For this review, use the dimensioned drawing (mm, ordinates from the lowest corner) and the shaded views. A direction names the side the tool comes from. Coordinates: 2 decimals unless noted, no trailing zeros. Loops run counter-clockwise (first coordinate to the right, second up) from the corner with the lowest first, then second, coordinate; pieces in that order, holes last. Notation, with made-up numbers: (-14, 67.25) - (26, 67.25) arc R27 cw to (26, 88.25) - close; hole circle Ø1 at (58, 71.25). An arc over 180 degrees is marked (long way). Answer in a Markdown table with one row per item. Add a question column.
(1) Mouldability with a two-part tool opening along Z and no side actions: class the marked faces 1, 2 and 3 as +Z half, -Z half, draft (parallel to the pull), parting line (faces both ways), or undercut.
(2) We need section B-B on x = 19.45. Write out the cut boundary in (y, z), plus the area to 3 significant figures.
(3) Machinability: for the marked faces 4, 5 and 6, which of the approach directions +Z, -Z, +X, -X, +Y, -Y give a long, thin tool a straight path to every point of the face, cutting with its end or side? Answer none if there is none.
(4) We need section C-C on z = 17.5. Write out the cut boundary in (x, y), plus the area to 3 significant figures.
(5) For P1, Ø1.7, axis at x = 10, z = 17.5, coming from the +Y side; P2, Ø10, axis at x = 24, z = 12, coming from the -Y side, all flat-tipped, find the tip position at first contact; note any pin that passes through.
(6) For line 1 along X through (y, z) = (4.5, 17.5); line 2 along Z through (x, y) = (3, 3.5); line 3 along Z through (x, y) = (9.75, 4), list the stretches that pass through material, from the lowest coordinate up.
(7) We need section D-D on x = 5.5. Write out the cut boundary in (y, z).
(8) We need section A-A on y = 5.25. Write out the cut boundary in (x, z), plus the area to 3 significant figures.
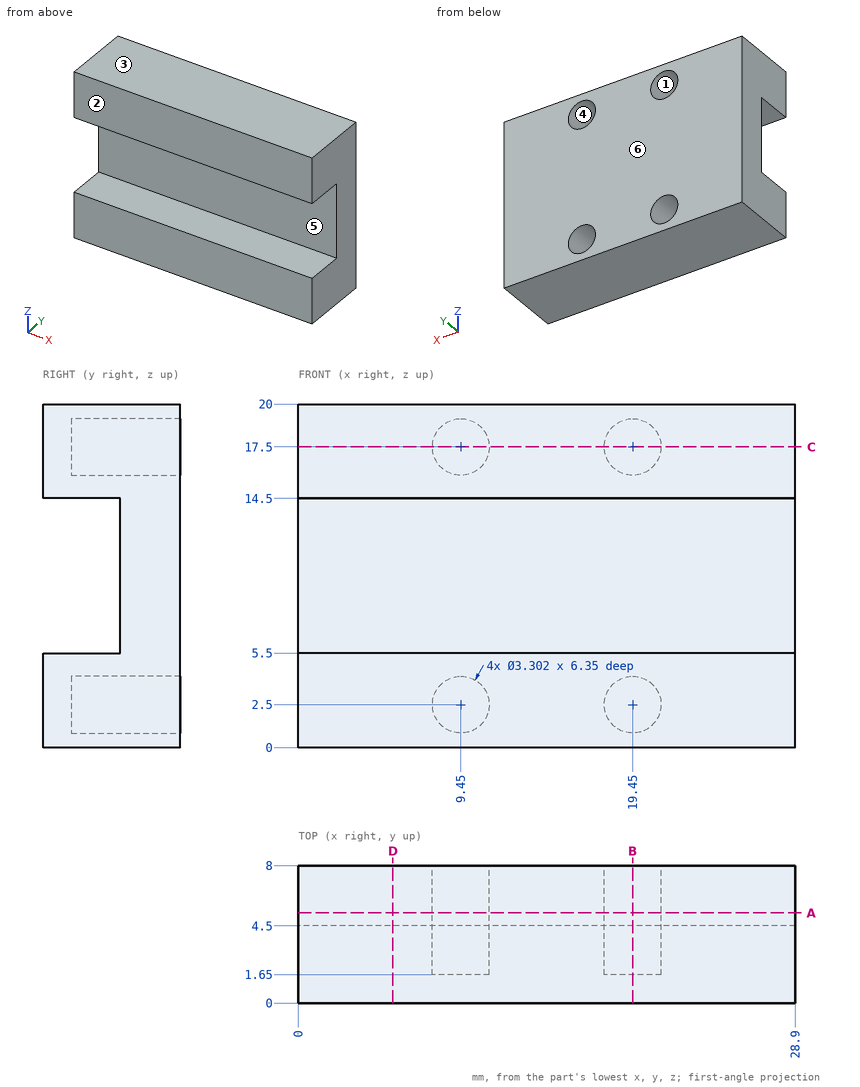
Outcome:
| question | item | result |
|---|---|---|
| 1 | face 1 | undercut |
| 1 | face 2 | draft |
| 1 | face 3 | +Z half |
| 2 | outline | (0, 0) - (8, 0) - (8, 0.85) - (1.65, 0.85) - (1.65, 4.15) - (8, 4.15) - (8, 15.85) - (1.65, 15.85) - (1.65, 19.15) - (8, 19.15) - (8, 20) - (0, 20) - (0, 14.5) - (4.5, 14.5) - (4.5, 5.5) - (0, 5.5) - close |
| 2 | area | 77.6 mm² |
| 3 | face 4 | +Y |
| 3 | face 5 | +X, -X, -Y |
| 3 | face 6 | +Z, -Z, +X, -X, +Y |
| 4 | outline | (0, 0) - (28.9, 0) - (28.9, 8) - (21.1, 8) - (21.1, 1.65) - (17.8, 1.65) - (17.8, 8) - (11.1, 8) - (11.1, 1.65) - (7.8, 1.65) - (7.8, 8) - (0, 8) - close |
| 4 | area | 189 mm² |
| 5 | P1 | y = 1.65 |
| 5 | P2 | y = 0 |
| 6 | line 1 | 0 to 7.8, 11.1 to 17.8, 21.1 to 28.9 |
| 6 | line 2 | 0 to 5.5, 14.5 to 20 |
| 6 | line 3 | 0 to 0.88, 4.12 to 5.5, 14.5 to 15.88, 19.12 to 20 |
| 7 | outline | (0, 0) - (8, 0) - (8, 20) - (0, 20) - (0, 14.5) - (4.5, 14.5) - (4.5, 5.5) - (0, 5.5) - close |
| 8 | outline | (0, 0) - (28.9, 0) - (28.9, 20) - (0, 20) - close; hole circle Ø3.3 at (9.45, 2.5); hole circle Ø3.3 at (9.45, 17.5); hole circle Ø3.3 at (19.45, 2.5); hole circle Ø3.3 at (19.45, 17.5) |
| 8 | area | 544 mm² |
